```python
from build123d import *

# Parameters (mm, degrees)
EXTRUDE_1_DEPTH     = 5
SKETCH_2_W          = 34
SKETCH_2_H          = 34
EXTRUDE_2_DEPTH     = 2
SKETCH_3_W          = 30.1
SKETCH_3_H          = 30.1
CUT_EXTRUDE_2_DEPTH = 2.08
CHAMFER_1_SIZE      = 1
FILLET_2_R          = 1


with BuildPart() as part:
    # 草图1 → 凸台-拉伸1 (new body)
    with BuildSketch(Plane(origin=(0, 0, 0), x_dir=(1, 0, 0), z_dir=(0, 1, 0))):
        Polygon((0, 10), (5, 10), (5, 22), (39, 22), (39, -12), (5, -12), (5, 0), (0, 0), align=None)
    extrude(amount=EXTRUDE_1_DEPTH)

    # 草图2 → 凸台-拉伸2 (add)
    with BuildSketch(Plane(origin=(0, 5, 0), x_dir=(1, 0, 0), z_dir=(0, 1, 0))):
        with Locations((22, 5)):
            Rectangle(SKETCH_2_W, SKETCH_2_H)
    extrude(amount=EXTRUDE_2_DEPTH)

    # 草图3 → 切除-拉伸2 (cut)
    with BuildSketch(Plane(origin=(0, 7, 0), x_dir=(1, 0, 0), z_dir=(0, 1, 0))):
        with Locations((22.05, 4.95)):
            Rectangle(SKETCH_3_W, SKETCH_3_H)
    extrude(amount=-CUT_EXTRUDE_2_DEPTH, mode=Mode.SUBTRACT)

    # 倒角1
    chamfer_1_edges = [part.edges().sort_by_distance(p)[0] for p in [
        (22.05, 7, -20),
        (37.1, 7, -4.95),
        (22.05, 7, 10.1),
        (7, 7, -4.95),
    ]]
    chamfer(chamfer_1_edges, length=CHAMFER_1_SIZE)

    # 圆角2
    fillet_2_edges = [part.edges().sort_by_distance(p)[0] for p in [
        (39, 3.5, 12),
        (39, 3.5, -22),
        (5, 3.5, -22),
        (22, 0, 12),
        (39, 0, -5),
        (22, 0, -22),
    ]]
    fillet(fillet_2_edges, radius=FILLET_2_R)


solid = part.part
```
Geometry check sheet. Reference: the model listing, model coordinates, mm. A direction names the side the tool comes from. Round coordinates to 2 decimals unless told otherwise and drop trailing zeros. Order: outer loops, then holes, each group sorted by start corner. A loop starts at its lowest first (then second) coordinate and runs counter-clockwise, first axis right, second up. Notation, with made-up numbers: (13, -15) - (49, -15) arc R24 ccw to (49, 12) - close; hole circle Ø6 at (84, -37). An arc over 180 degrees is marked (long way). Use a Markdown table: item, result. Add a question column.
1) Mould release check, pull along Z, two halves, no side actions. Record for faces 4 (the flat face through (21, 4, 12)), 5 (the flat face through (7, 5.5, -4.7)), 6 (the flat face through (20.7, 7, 11.3)): released by +Z, released by -Z, zero draft, split by the parting line, or undercut.
2) Thickness scan on line 1 along Z through (x, y) = (10, 5.5); line 2 along X through (y, z) = (6, -1); line 3 along Y through (x, z) = (35, -9). Record the ranges inside material, lowest first.
3) Gauge pin test, flat ends, axial feed: P1, Ø1.5, axis at x = 2, y = 2.5, coming from the -Z side; P2, Ø1.5, axis at x = 2.5, z = -5, coming from the +Y side. Record the tip position at first contact, or that the pin passes through.
4) Section check A-A (y = 5.5). Record the cut outline in (x, z), then the cut area to 3 significant figures.
5) Set-up check for faces 1 (the flat face through (3, 2, 0)), 2 (the flat face through (2, 2, -10)), 3 (the flat face through (3, 5, -5)): record each of +Z, -Z, +X, -X, +Y, -Y from which the full face is reachable in a straight line by a thin tool's end or side.
6) Section check D-D (y = 3.25). Record the cut outline in (x, z).
7) Section check C-C (z = -3). Record the cut outline in (x, y), then the cut area to 3 significant figures.
8) Section check B-B (x = 14). Record the cut outline in (y, z).
Established:
| question | item | result |
|---|---|---|
| 1 | face 4 | released by +Z |
| 1 | face 5 | undercut |
| 1 | face 6 | zero draft |
| 2 | line 1 | -22 to -20, 10.1 to 12 |
| 2 | line 2 | 5 to 7, 37.1 to 39 |
| 2 | line 3 | 0 to 4.92 |
| 3 | P1 | z = -10 |
| 3 | P2 | y = 5 |
| 4 | outline | (5, -21) arc R1 ccw to (6, -22) - (38, -22) arc R1 ccw to (39, -21) - (39, 11) arc R1 ccw to (38, 12) - (5, 12) - close; hole (7, -20) - (37.1, -20) - (37.1, 10.1) - (7, 10.1) - close |
| 4 | area | 249 mm2 |
| 5 | face 1 | +Z, -X, +Y, -Y |
| 5 | face 2 | -Z, -X, +Y, -Y |
| 5 | face 3 | +Z, -Z, -X, +Y |
| 6 | outline | (0, -10) - (5, -10) - (5, -21) arc R1 ccw to (6, -22) - (38, -22) arc R1 ccw to (39, -21) - (39, 11) arc R1 ccw to (38, 12) - (5, 12) - (5, 0) - (0, 0) - close |
| 7 | outline | (0, 0) - (38, 0) arc R1 ccw to (39, 1) - (39, 7) - (38.1, 7) - (37.1, 6) - (37.1, 4.92) - (7, 4.92) - (7, 6) - (6, 7) - (5, 7) - (5, 5) - (0, 5) - close |
| 7 | area | 199 mm2 |
| 8 | outline | (0, -21) arc R1 ccw to (1, -22) - (7, -22) - (7, -21) - (6, -20) - (4.92, -20) - (4.92, 10.1) - (6, 10.1) - (7, 11.1) - (7, 12) - (1, 12) arc R1 ccw to (0, 11) - close |
